```python
from build123d import *

# Parameters (mm, degrees)
F1_DEPTH = 12.6
F2_R     = 1.75
F3_DEPTH = 2
F4_R     = 2.3
F5_DEPTH = 3.2
F6_R     = 5
F7_W     = 5.6
F7_H     = 2
F8_DEPTH = 2
F9_R     = 0.5


with BuildPart() as f1:
    # F0 (on Front) → F1 (new body)
    with BuildSketch(Plane.XZ):
        Polygon((-4.85, 16), (0, 16), (0, 0), (22.8, 0), (22.8, 16), (27.65, 16), (27.65, 18), (22.65, 18), (22.65, 22.5), (14.568375, 22.5), (14.568375, 26.5), (1.7551, 26.5), (1.7551, 22.5), (0, 22.5), (0, 18), (-4.85, 18), align=None)
    extrude(amount=F1_DEPTH)

    # F2 (on face) → F3 (cut, through all)
    with BuildSketch(Plane.XY.offset(18)):
        with Locations((-2.4, -6.3)):
            Circle(F2_R)
        with Locations((25.2, -6.3)):
            Circle(F2_R)
    extrude(amount=-F3_DEPTH, mode=Mode.SUBTRACT)

    # F4 (on face) → F5 (join)
    with BuildSketch(Plane.XY.offset(26.5)):
        with Locations((5.9, -6.3)):
            Circle(F4_R)
    extrude(amount=F5_DEPTH)

    # F6
    f6_edges = [f1.edges().sort_by_distance(p)[0] for p in [
        (14.568375, 0, 24.5),
        (14.568375, -12.6, 24.5),
        (1.7551, -12.6, 24.5),
        (1.7551, 0, 24.5),
    ]]
    fillet(f6_edges, radius=F6_R)

    # F7 (on face) → F8 (join)
    with BuildSketch(Plane(origin=(0, 0, 0), x_dir=(0, -1, 0), z_dir=(-1, 0, 0))):
        with Locations((5.8, 5)):
            Rectangle(F7_W, F7_H)
    extrude(amount=F8_DEPTH)

    # F9
    f9_edges = [f1.edges().sort_by_distance(p)[0] for p in [
        (-1, -8.6, 6),
        (-1, -3, 6),
        (-1, -3, 4),
        (-1, -8.6, 4),
    ]]
    fillet(f9_edges, radius=F9_R)


solid = f1.part
```
Geometry: final body of the model. Coordinates: model frame, mm. A direction names the side the tool comes from. Round coordinates to 2 decimals unless told otherwise and drop trailing zeros. Write each loop counter-clockwise with the first axis right and the second up, starting at its lowest first coordinate (ties: lowest second). Pieces come first, ordered by that corner, then holes.
Item 1: Mould query, pull axis Y, two halves, no side actions, for faces 4 (the face through (13.065, -1.426, 24.528)), 5 (the face through (-2.78, -8.01, 17.01)), 6 (the face through (6, -6, 29.7)). Classes: +Y half, -Y half, draft (parallel to the pull), parting line (faces both ways), or undercut.
Item 2: Section query D-D (x = 5.9). Return loops of the section in (y, z).
Item 3: Pin query (flat end, axial travel): P1, Ø4, axis at y = -7, z = 9, coming from the +X side; P2, Ø1.3, axis at y = -7, z = 19.5, coming from the -X side; P3, Ø2, axis at x = 2.5, y = -6.5, coming from the +Z side. Return the tip coordinate at first contact, or that it passes through.
Item 4: Material intervals for L1, parallel to Y at x = -2.4, z = 17.4; L2, parallel to Z at x = 23.5, y = -8.5; L3, parallel to X at y = -11.5, z = 21.75, sorted ascending.
Item 5: Section query B-B (y = -6.3). Give the number of separate pieces and of enclosed holes in the cut face, plus the area to 3 significant figures.
Item 6: Section query A-A (x = -2.4). Return loops of the section in (y, z).
Item 7: Section query C-C (z = 23.5). Return loops of the section in (x, y), plus the area to 3 significant figures.
Item 8: Set-up query: faces 1 (the face through (13.065, -11.174, 24.528)), 2 (the face through (22.65, -6, 20)), 3 (the face through (1, -6, 22.5)). Return all of +Z, -Z, +X, -X, +Y, -Y with unobstructed straight access to the full face (end or side cutting, diameter ignored); none if empty.
Completed:
1. face 4: +Y half
1. face 5: undercut
1. face 6: draft
2. outline: (-12.6, 0) - (0, 0) - (0, 22.5) - (-0.07, 22.5) - (-0.07, 26.5) - (-4, 26.5) - (-4, 29.7) - (-8.6, 29.7) - (-8.6, 26.5) - (-12.53, 26.5) - (-12.53, 22.5) - (-12.6, 22.5) - close
3. P1: stops at x = 22.8
3. P2: stops at x = 0
3. P3: stops at z = 26.5
4. L1: y = -12.6 to -8.05, -4.55 to 0
4. L2: z = 16 to 18
4. L3: x = 0 to 22.65
5. separate pieces: 3
5. enclosed holes: 0
5. area: 588 mm2
6. outline: (-12.6, 16) - (-8.05, 16) - (-8.05, 18) - (-12.6, 18) - close; (-4.55, 16) - (0, 16) - (0, 18) - (-4.55, 18) - close
7. outline: (1.76, -7.6) arc R5 ccw to (6.76, -12.6) - (9.57, -12.6) arc R5 ccw to (14.57, -7.6) - (14.57, -5) arc R5 ccw to (9.57, 0) - (6.76, 0) arc R5 ccw to (1.76, -5) - close
7. area: 140 mm2
8. face 1: +Z, +X, -Y
8. face 2: +Z, +X, +Y, -Y
8. face 3: +Z, -X
